```python
from build123d import *

# Parameters (mm, degrees)
F0_R      = 4.191
F1_DEPTH  = 73.66
F2_R      = 4.191
F3_DEPTH  = 8.382
F4_R      = 4.19099
F5_R      = 6.35
F6_DEPTH  = 1.27
F7_R      = 29.9024876922
F8_DEPTH  = 73.66
F9_R      = 1.905
F10_DEPTH = 12.7


# Not quite as in the source:
# - a fillet or chamfer is up to 0.001 mm smaller than in the source, because OpenCascade refuses the exact size


with BuildPart() as f1:
    # F0 (on Top) → F1 (new body)
    with BuildSketch(Plane.XY):
        Circle(F0_R)
    extrude(amount=F1_DEPTH)



with BuildPart() as f3:
    # F2 (on face) → F3 (new body)
    with BuildSketch(Plane.XY.offset(73.66)):
        Circle(F2_R)
    extrude(amount=F3_DEPTH)

    # F4 (radius 4.191 in the source; OpenCascade refuses exactly that, so slightly less here)
    f4_edges = [f3.edges().sort_by_distance(p)[0] for p in [
        (-4.191, 0, 73.66),
        (-4.191, 0, 82.042),
    ]]
    fillet(f4_edges, radius=F4_R)


with BuildPart() as f1_1:
    add(f1.part)

    add(f3.part)  # F6 merges F3
    # F5 (on face) → F6 (join)
    with BuildSketch(Plane.XY.offset(73.66)):
        Circle(F5_R)
    extrude(amount=F6_DEPTH)

    # F7 (on face) → F8 (cut)
    with BuildSketch(Plane(origin=(0, 0, 0), x_dir=(1, 0, 0), z_dir=(0, 0, -1))):
        Circle(F7_R)
    extrude(amount=-F8_DEPTH, mode=Mode.SUBTRACT)

    # F9 (on face) → F10 (join)
    with BuildSketch(Plane(origin=(0, 0, 73.66), x_dir=(1, 0, 0), z_dir=(0, 0, -1))):
        Circle(F9_R)
    extrude(amount=F10_DEPTH)


solid = f1_1.part
```
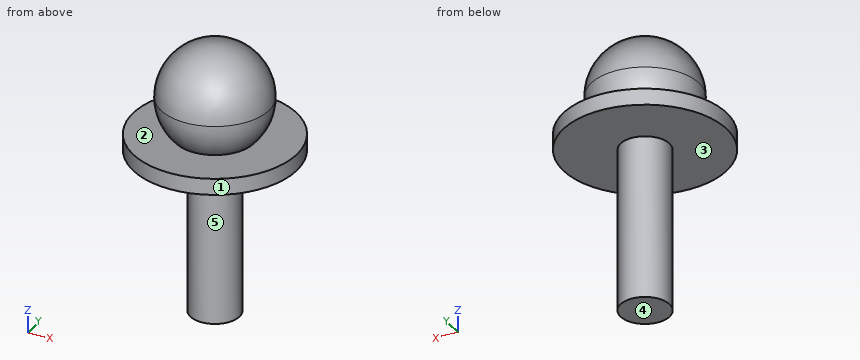
Input: part model. Units: mm. Frame: model coordinates. Face numbers are marked on the shaded views. A direction names the side the tool comes from. Coordinates: 2 decimals unless noted, no trailing zeros. Write each loop counter-clockwise with the first axis right and the second up, starting at its lowest first coordinate (ties: lowest second). Pieces come first, ordered by that corner, then holes. Notation, with made-up numbers: (41.25, 29.5) -> (82.25, 29.5) arc R27 ccw to (82.25, 58.5) -> close; hole circle Ø6 at (5.5, 61.5). An arc over 180 degrees is marked (long way). Answer as a JSON object with one key per item and string values.
1. Access query for the marked faces 4 and 5. Directions: +Z, -Z, +X, -X, +Y, -Y. A direction counts if a zero-diameter tool reaches every point of the face in a straight line with its end or side. Return the directions, or none.
Result set:
{"face 4": "-Z, +X, -X, +Y, -Y", "face 5": "-Z"}
2. Material intervals for line 1 (Y direction, x = 0, z = 72) (3 decimals); line 2 (Z direction, x = 1.75, y = 3); line 3 (Z direction, x = 4.25, y = -1.75), sorted ascending. Write a range as from..to.
Result set:
{"line 1": "y = -1.905..1.905", "line 2": "z = 73.66..74.93, 75.51..80.2", "line 3": "z = 73.66..74.93"}
3. Section A-A on z = 68. Return the cut outline in (x, y) (3 decimals), then the cut area to 3 significant figures.
Result set:
{"outline": "circle Ø3.81 at (0, 0)", "area": "11.4 mm2"}
4. Section B-B on y = 5.5. Return the cut outline in (x, z), then the cut area to 3 significant figures.
Result set:
{"outline": "(-3.17, 73.66) -> (3.17, 73.66) -> (3.17, 74.93) -> (-3.17, 74.93) -> close", "area": "8.06 mm2"}
5. First-contact query: P1, Ø2, axis at y = -3.5, z = 64.5, coming from the -X side; P2, Ø3, axis at y = -3, z = 72, coming from the -X side; P3, Ø6, axis at x = -2.5, z = 65, coming from the +Y side (3 decimals); P4, Ø3, axis at x = 4, y = -0.5, coming from the -Z side. Flat tips, straight axial feed; report the tip coordinate or a pass-through.
Result set:
{"P1": "passes through", "P2": "stops at x = -1.17", "P3": "stops at y = 1.905", "P4": "stops at z = 73.66"}
6. Mould query, pull axis Z, two halves, no side actions, for the marked faces 1, 2 and 3. Classes: released by +Z, released by -Z, zero draft, split by the parting line, or undercut.
Result set:
{"face 1": "zero draft", "face 2": "undercut", "face 3": "released by -Z"}
